```python
from build123d import *

# Parameters (mm, degrees)
AUFSATZ_LINEAR_AUSTRAGEN1_DEPTH      = 150
SCHNITT_LINEAR_AUSTRAGEN2_DEPTH      = 658.647321898
SCHNITT_LINEAR_AUSTRAGEN2_DEPTH_BACK = 658.647321898
SCHNITT_LINEAR_AUSTRAGEN7_REACH      = 928.607
SCHNITT_LINEAR_AUSTRAGEN7_END_RADIUS = 10
SCHNITT_LINEAR_AUSTRAGEN8_DEPTH      = 180
AUFSATZ_LINEAR_AUSTRAGEN2_DEPTH      = 150
SKIZZE15_W                           = 1390.722154613
SKIZZE15_H                           = 110
SCHNITT_LINEAR_AUSTRAGEN16_DEPTH     = 1000
SCHNITT_LINEAR_AUSTRAGEN22_DEPTH     = 200
SCHNITT_LINEAR_AUSTRAGEN27_DEPTH     = 120
SKIZZE2_R                            = 5
SCHNITT_LINEAR_AUSTRAGEN28_DEPTH     = 10
AUFSATZ_LINEAR_AUSTRAGEN3_DEPTH      = 40
SCHNITT_LINEAR_AUSTRAGEN29_DEPTH     = 200
SCHNITT_LINEAR_START                 = 300
SCHNITT_LINEAR_AUSTRAGEN30_DEPTH     = 300


with BuildPart() as part:
    # Skizze1 → Aufsatz-Linear austragen1 (new body)
    with BuildSketch(Plane.XY):
        with BuildLine():
            Line((150, 600), (-150, 600))
            ThreePointArc((-150, 600), (-353.150600634, 544.571956871), (-500, 393.64916731))
            Line((-500, 393.64916731), (-500, 200))
            Line((-500, 200), (-350, 200))
            ThreePointArc((-350, 200), (-291.421356237, 341.421356237), (-150, 400))
            Line((-150, 400), (150, 400))
            ThreePointArc((150, 400), (291.421356237, 341.421356237), (350, 200))
            Line((350, 200), (500, 200))
            Line((500, 200), (500, 393.64916731))
            ThreePointArc((500, 393.64916731), (353.150600634, 544.571956871), (150, 600))
        make_face()
    extrude(amount=AUFSATZ_LINEAR_AUSTRAGEN1_DEPTH)

    # Skizze4 → Schnitt-Linear austragen2 (cut, two sides: drawn at the far end of the back side and taken through both)
    with BuildSketch(Plane(origin=(0, 600, 0), x_dir=(1, 0, 0), z_dir=(0, 1, 0)).offset(-SCHNITT_LINEAR_AUSTRAGEN2_DEPTH_BACK)):
        with BuildLine():
            Line((-310, -120), (-190, -120))
            ThreePointArc((-190, -120), (-180, -130), (-190, -140))
            Line((-190, -140), (-310, -140))
            ThreePointArc((-310, -140), (-320, -130), (-310, -120))
        make_face()
        with BuildLine():
            Line((190, -120), (310, -120))
            ThreePointArc((310, -120), (320, -130), (310, -140))
            Line((310, -140), (190, -140))
            ThreePointArc((190, -140), (180, -130), (190, -120))
        make_face()
    extrude(amount=SCHNITT_LINEAR_AUSTRAGEN2_DEPTH + SCHNITT_LINEAR_AUSTRAGEN2_DEPTH_BACK, mode=Mode.SUBTRACT)

    # Schnitt-Linear austragen7: up to this cylinder (the profile starts outside it)
    schnitt_linear_austragen7_end = Plane(origin=(190, 420, 130), z_dir=(0, 1, 0)) * Cylinder(SCHNITT_LINEAR_AUSTRAGEN7_END_RADIUS, 1878.214, mode=Mode.PRIVATE)
    # Skizze5 → Schnitt-Linear austragen7 (cut, up to the surface)
    with BuildSketch(Plane.ZY.offset(190), mode=Mode.PRIVATE) as schnitt_linear_austragen7_sk1:
        with BuildLine():
            Line((140, 425), (140, 415))
            ThreePointArc((140, 415), (130, 405), (120, 415))
            Line((120, 415), (120, 425))
            ThreePointArc((120, 425), (130, 435), (140, 425))
        make_face()
    schnitt_linear_austragen7_tool1 = extrude(schnitt_linear_austragen7_sk1.sketch, amount=-SCHNITT_LINEAR_AUSTRAGEN7_REACH, mode=Mode.PRIVATE) - schnitt_linear_austragen7_end
    add(schnitt_linear_austragen7_tool1.solids().sort_by_distance((-190, 420, 130))[0], mode=Mode.SUBTRACT)

    # Skizze3 → Schnitt-Linear austragen8 (cut)
    with BuildSketch(Plane(origin=(0, 600, 0), x_dir=(1, 0, 0), z_dir=(0, 1, 0))):
        with BuildLine():
            Line((-25, -120), (25, -120))
            ThreePointArc((25, -120), (35, -130), (25, -140))
            Line((25, -140), (-25, -140))
            ThreePointArc((-25, -140), (-35, -130), (-25, -120))
        make_face()
    extrude(amount=-SCHNITT_LINEAR_AUSTRAGEN8_DEPTH, mode=Mode.SUBTRACT)

    # Skizze11 → Aufsatz-Linear austragen2 (add)
    with BuildSketch(Plane.XY):
        Polygon((356, 200), (350, 200), (350, 194), (360, 194), (360, 197), (356, 197), align=None)
        Polygon((390, 194), (390, 200), (384, 200), (384, 197), (380, 197), (380, 194), align=None)
    extrude(amount=AUFSATZ_LINEAR_AUSTRAGEN2_DEPTH)

    # Skizze15 → Schnitt-Linear austragen16 (cut)
    with BuildSketch(Plane(origin=(0, 600, 0), x_dir=(1, 0, 0), z_dir=(0, 1, 0))):
        with Locations((37.447933541, -55)):
            Rectangle(SKIZZE15_W, SKIZZE15_H)
    extrude(amount=-SCHNITT_LINEAR_AUSTRAGEN16_DEPTH, mode=Mode.SUBTRACT)

    # Skizze17 → Schnitt-Linear austragen22 (cut)
    with BuildSketch(Plane.XY.offset(150)):
        with BuildLine():
            ThreePointArc((-728.904569039, 200), (-39.53876737, 889.365801669), (649.827034299, 200))
            Line((649.827034299, 200), (390, 200))
            ThreePointArc((390, 200), (319.705627485, 369.705627485), (150, 440))
            Line((150, 440), (-150, 440))
            ThreePointArc((-150, 440), (-319.705627485, 369.705627485), (-390, 200))
            Line((-390, 200), (-728.904569039, 200))
        make_face()
    extrude(amount=-SCHNITT_LINEAR_AUSTRAGEN22_DEPTH, mode=Mode.SUBTRACT)

    # Skizze9 → Schnitt-Linear austragen27 (cut)
    with BuildSketch(Plane(origin=(0, 0, 0), x_dir=(-1, 0, 0), z_dir=(0, 0, -1))):
        Polygon((-12.979274058, 426.5), (-10.958548116, 430), (-12.979274058, 433.5), (-17.020725942, 433.5), (-19.041451884, 430), (-17.020725942, 426.5), align=None)
        Polygon((17.020725942, 426.5), (12.979274058, 426.5), (10.958548116, 430), (12.979274058, 433.5), (17.020725942, 433.5), (19.041451884, 430), align=None)
        Polygon((-12.979274058, 406.5), (-10.958548116, 410), (-12.979274058, 413.5), (-17.020725942, 413.5), (-19.041451884, 410), (-17.020725942, 406.5), align=None)
        Polygon((17.020725942, 406.5), (12.979274058, 406.5), (10.958548116, 410), (12.979274058, 413.5), (17.020725942, 413.5), (19.041451884, 410), align=None)
    extrude(amount=-SCHNITT_LINEAR_AUSTRAGEN27_DEPTH, mode=Mode.SUBTRACT)

    # Skizze2 → Schnitt-Linear austragen28 (cut)
    with BuildSketch(Plane.XZ.offset(-200)):
        with Locations(Location((-370, 130, 0), (0, 0, 270))):
            Circle(SKIZZE2_R)
        with Locations(Location((370, 130, 0), (0, 0, 270))):
            Circle(SKIZZE2_R)
    extrude(amount=-SCHNITT_LINEAR_AUSTRAGEN28_DEPTH, mode=Mode.SUBTRACT)

    # Skizze21 → Aufsatz-Linear austragen3 (add)
    with BuildSketch(Plane.XY.offset(150)):
        Polygon((-384, 200), (-390, 200), (-390, 194), (-380, 194), (-380, 197), (-384, 197), align=None)
        Polygon((-350, 194), (-350, 200), (-356, 200), (-356, 197), (-360, 197), (-360, 194), align=None)
    extrude(amount=-AUFSATZ_LINEAR_AUSTRAGEN3_DEPTH)

    # Skizze22 → Schnitt-Linear austragen29 (cut)
    with BuildSketch(Plane.ZY.offset(190)):
        with BuildLine():
            Line((140, 270), (140, 250))
            ThreePointArc((140, 250), (130, 240), (120, 250))
            Line((120, 250), (120, 270))
            ThreePointArc((120, 270), (130, 280), (140, 270))
        make_face()
    extrude(amount=SCHNITT_LINEAR_AUSTRAGEN29_DEPTH, mode=Mode.SUBTRACT)

    # Skizze23 → Schnitt-Linear austragen30 (cut)
    with BuildSketch(Plane(origin=(150, 0, 0), x_dir=(0, 0, -1), z_dir=(1, 0, 0)).offset(SCHNITT_LINEAR_START)):
        with BuildLine():
            Line((-120, 270), (-120, 250))
            ThreePointArc((-120, 250), (-130, 240), (-140, 250))
            Line((-140, 250), (-140, 270))
            ThreePointArc((-140, 270), (-130, 280), (-120, 270))
        make_face()
    extrude(amount=-SCHNITT_LINEAR_AUSTRAGEN30_DEPTH, mode=Mode.SUBTRACT)


solid = part.part
```
Could you check a few things on this model? Use its own coordinates, in mm. A direction names the side the tool comes from. Round coordinates to 2 decimals unless told otherwise and drop trailing zeros. Loops run counter-clockwise (first coordinate to the right, second up) from the corner with the lowest first, then second, coordinate; pieces in that order, holes last.
Q1. Thinking about a two-plate mould opening in Y: for faces 6 (the cylindrical face through (-3, 405, 130)), 7 (the flat face through (-2, 400, 130)), 8 (the cylindrical face through (320, 342, 130)), which applies, pulls with the +Y half, pulls with the -Y half, needs draft (parallel to the pull), parting line crosses it, or undercut?
Q2. I want a section at C-C (x = -299.5). Write out the boundary of the cut face in (y, z), and give its area (3 significant figures).
Q3. I want a section at B-B (x = 203.5). Write out the boundary of the cut face in (y, z).
Q4. Please list where these lines run through material, in increasing order: L1, parallel to X at y = 202.75, z = 130; L2, parallel to X at y = 205.75, z = 130; L3, parallel to Z at x = -370, y = 206.75.
Q5. For P1, Ø5, axis at y = 233, z = 145, coming from the +X side; P2, Ø4.5, axis at x = -15, z = 116.5, coming from the -Y side; P3, Ø6, axis at y = 315.5, z = 121.5, coming from the +X side, each with a flat end and sliding along its axis, tell me the tip position at first contact or that it passes through.
Q6. I want a section at A-A (y = 350.5). Write out the boundary of the cut face in (x, z), and give its area (3 significant figures).
Q7. On a 3-axis mill with a long thin cutter (end or side, diameter ignored), from which of +Z, -Z, +X, -X, +Y, -Y can I reach the whole of each face in a straight line? I mean faces 1 (the cylindrical face through (-317.83, 371.56, 139.17)), 2 (the cylindrical face through (-109, 435, 130)), 3 (the cylindrical face through (-35, 436, 130)), 4 (the flat face through (-373, 200, 125)), 5 (the cylindrical face through (-292.968, 339.858, 116.387)). Say none if no direction works.
Answer below:
1. face 6: undercut
1. face 7: pulls with the -Y half
1. face 8: needs draft
2. outline: (332.85, 110) - (387.75, 110) - (387.75, 120) - (332.85, 120) - close; (332.85, 140) - (387.75, 140) - (387.75, 150) - (332.85, 150) - close
2. area: 1,100 mm2
3. outline: (392.71, 110) - (433.96, 110) - (433.96, 120) - (392.71, 120) - close; (392.71, 140) - (433.96, 140) - (433.96, 150) - (392.71, 150) - close
4. L1: x = -389.98 to -375, -365 to -349.98, 349.98 to 365, 375 to 389.98
4. L2: x = -389.93 to -375, -365 to -349.92, 349.92 to 365, 375 to 389.93
4. L3: z = 110 to 125, 135 to 150
5. P1: stops at x = 388.05
5. P2: stops at y = 400
5. P3: stops at x = 362
6. outline: (-336.95, 110) - (-281.72, 110) - (-281.72, 120) - (-310, 120) arc R10 cw to (-310, 140) - (-281.72, 140) - (-281.72, 150) - (-336.95, 150) - close; (281.72, 110) - (336.95, 110) - (336.95, 150) - (281.72, 150) - (281.72, 140) - (310, 140) arc R10 cw to (310, 120) - (281.72, 120) - close
6. area: 2,970 mm2
7. face 1: +Z, -Z, -X, +Y
7. face 2: +X, -X
7. face 3: +Y
7. face 4: +Z, -Z
7. face 5: +Z, -Z, -Y
